```python
from build123d import *

# Parameters (mm, degrees)
SKETCH2_R           = 25
BOSS_EXTRUDE2_DEPTH = 10
SKETCH3_W           = 10
SKETCH3_H           = 20
BOSS_EXTRUDE3_DEPTH = 25
SKETCH4_R           = 5
CUT_EXTRUDE1_DEPTH  = 20
FILLET1_R           = 10
SKETCH5_R           = 17.5
SKETCH5_R_2         = 12.5
BOSS_EXTRUDE4_DEPTH = 150


with BuildPart() as part:
    # Sketch2 → Boss-Extrude2 (new body)
    with BuildSketch(Plane.XY):
        Circle(SKETCH2_R)
    extrude(amount=BOSS_EXTRUDE2_DEPTH)

    # Sketch3 → Boss-Extrude3 (add)
    with BuildSketch(Plane.XY.offset(10)):
        Rectangle(SKETCH3_W, SKETCH3_H)
    extrude(amount=BOSS_EXTRUDE3_DEPTH)

    # Sketch4 → Cut-Extrude1 (cut)
    with BuildSketch(Plane.ZY.offset(5)):
        with Locations(Location((25, 0, 0), (0, 0, 270))):
            Circle(SKETCH4_R)
    extrude(amount=-CUT_EXTRUDE1_DEPTH, mode=Mode.SUBTRACT)

    # Fillet1
    fillet1_edges = [part.edges().sort_by_distance(p)[0] for p in [
        (0, -10, 35),
        (0, 10, 35),
    ]]
    fillet(fillet1_edges, radius=FILLET1_R - 0.0001)  # a hair under: the kernel refuses the full size

    # Sketch5 → Boss-Extrude4 (add)
    with BuildSketch(Plane(origin=(0, 0, 0), x_dir=(-1, 0, 0), z_dir=(0, 0, -1))):
        with Locations(Location((0, 0, 0), (0, 0, 180))):
            Circle(SKETCH5_R)
        Circle(SKETCH5_R_2, mode=Mode.SUBTRACT)
    extrude(amount=BOSS_EXTRUDE4_DEPTH)


solid = part.part
```
For this review, take the finished solid that the model builds, in its own axes (mm). A direction names the side the tool comes from. Coordinates: 2 decimals unless noted, no trailing zeros. Write each loop counter-clockwise with the first axis right and the second up, starting at its lowest first coordinate (ties: lowest second). Pieces come first, ordered by that corner, then holes.
(1) For pin 1 Ø1 at (y, z) = (-16.5, -130) entering from +X; pin 2 Ø3 at (x, y) = (18, -19.5) entering from -Z; pin 3 Ø5 at (x, z) = (1.5, 17.5) entering from -Y; pin 4 Ø25 at (x, y) = (1.5, -10.5) entering from +Z, all flat-tipped, find the tip position at first contact; note any pin that passes through.
(2) The part is to be moulded in two halves that separate along Y. For faces 1 (the face through (0, 0, 0)), 2 (the face through (5.2, 0.4, 10)), 3 (the face through (-0.07, 1.08, 20.12)), 4 (the face through (0.07, 7.15, 31.99)), say which applies: +Y half, -Y half, draft (parallel to the pull), parting line (faces both ways), or undercut.
(3) Add section D-D on x = -10.5. Give the boundary of the cut face in (y, z).
(4) Wall thickness on probe 1 along Z at (x, y) = (0, 0); probe 2 along Y at (x, z) = (0, -52); probe 3 along Z at (x, y) = (-18, -2): over which ranges is each line inside the solid? List them lowest first.
(5) Tool access review of faces 5 (the face through (0, 10, 17)), 6 (the face through (5, -0.1, 19.5)), 7 (the face through (-11.923, 3.755, -73.95)), 8 (the face through (0, -10, 17)): name each direction out of +Z, -Z, +X, -X, +Y, -Y from which nothing blocks a thin tool from reaching the whole face with its end or side.
(6) Add section B-B on y = 15.5. Give the boundary of the cut face in (x, z).
(7) Add section C-C on z = -83. Give the boundary of the cut face in (x, y), then the cut area to 3 significant figures.
Answer sheet:
1. pin 1: stops at x = 7.09
1. pin 2: passes through
1. pin 3: stops at y = -10
1. pin 4: stops at z = 35
2. face 1: undercut
2. face 2: draft
2. face 3: undercut
2. face 4: +Y half
3. outline: (-22.69, 0) - (-14, 0) - (-14, -150) - (-6.78, -150) - (-6.78, 0) - (6.78, 0) - (6.78, -150) - (14, -150) - (14, 0) - (22.69, 0) - (22.69, 10) - (-22.69, 10) - close
4. probe 1: z = 0 to 20, 30 to 35
4. probe 2: y = -17.5 to -12.5, 12.5 to 17.5
4. probe 3: z = 0 to 10
5. face 5: +Z, +X, -X, +Y
5. face 6: +Z, +X, +Y, -Y
5. face 7: -Z
5. face 8: +Z, +X, -X, -Y
6. outline: (-19.62, 0) - (-8.12, 0) - (-8.12, -150) - (8.12, -150) - (8.12, 0) - (19.62, 0) - (19.62, 10) - (-19.62, 10) - close
7. outline: circle Ø35 at (0, 0); hole circle Ø25 at (0, 0)
7. area: 471 mm2
